from build123d import *

# Parameters (mm, degrees)
SKETCH1_W                     = 32.5
SKETCH1_H                     = 40
BASE_DEPTH                    = 4
SKETCH4_R                     = 0.9
SCANNER_MOUNTING_HOLES_DEPTH  = 44.359687499
SKETCH6_W                     = 6
SKETCH6_H                     = 4.5
SERVO_MOUNTING_PLATFORM_DEPTH = 14
SERVO_MOUNTING_HOLES_REACH    = 51.46
SKETCH7_R                     = 0.9
FILLET1_R                     = 1


with BuildPart() as part:
    # Sketch1 → Base (new body)
    with BuildSketch(Plane(origin=(0, 0, 0), x_dir=(1, 0, 0), z_dir=(0, 1, 0))):
        with Locations((0, 20)):
            Rectangle(SKETCH1_W, SKETCH1_H)
    extrude(amount=BASE_DEPTH)

    # Sketch4 → Scanner Mounting Holes (cut, through all)
    with BuildSketch(Plane.XZ):
        with Locations(Location((-12.35, -6, 0), (0, 0, 270))):
            Circle(SKETCH4_R)
        with Locations(Location((-12.35, -32.4, 0), (0, 0, 270))):
            Circle(SKETCH4_R)
        with Locations(Location((12.35, -32.4, 0), (0, 0, 90))):
            Circle(SKETCH4_R)
        with Locations(Location((12.35, -6, 0), (0, 0, 90))):
            Circle(SKETCH4_R)
    extrude(amount=-SCANNER_MOUNTING_HOLES_DEPTH, mode=Mode.SUBTRACT)

    # Sketch6 → Servo Mounting Platform (add)
    with BuildSketch(Plane.XZ):
        with Locations((-6.25, -6)):
            Rectangle(SKETCH6_W, SKETCH6_H)
        with Locations((-6.25, -33.8)):
            Rectangle(SKETCH6_W, SKETCH6_H)
    extrude(amount=SERVO_MOUNTING_PLATFORM_DEPTH)

    # Sketch7 → Servo Mounting Holes (cut, up to next)
    with BuildSketch(Plane.ZY.offset(9.25), mode=Mode.PRIVATE) as servo_mounting_holes_sk1:
        with Locations((-33.8, -8)):
            Circle(SKETCH7_R)
    servo_mounting_holes_tool1 = extrude(servo_mounting_holes_sk1.sketch, amount=-SERVO_MOUNTING_HOLES_REACH, mode=Mode.PRIVATE) & part.part
    # Sketch7 → Servo Mounting Holes (cut, up to next)
    with BuildSketch(Plane.ZY.offset(9.25), mode=Mode.PRIVATE) as servo_mounting_holes_sk2:
        with Locations((-6, -8)):
            Circle(SKETCH7_R)
    servo_mounting_holes_tool2 = extrude(servo_mounting_holes_sk2.sketch, amount=-SERVO_MOUNTING_HOLES_REACH, mode=Mode.PRIVATE) & part.part
    add(servo_mounting_holes_tool1.solids().sort_by_distance((-9.25, -8, -33.8))[0], mode=Mode.SUBTRACT)
    add(servo_mounting_holes_tool2.solids().sort_by_distance((-9.25, -8, -6))[0], mode=Mode.SUBTRACT)

    # Fillet1
    fillet1_edges = [part.edges().sort_by_distance(p)[0] for p in [
        (16.25, 4, -20),
        (0, 4, -40),
        (-6.25, 0, -8.25),
        (-6.25, 0, -3.75),
        (-9.25, -14, -6),
        (-6.25, -14, -8.25),
        (-3.25, -14, -6),
        (-6.25, -14, -3.75),
        (-6.25, 0, -36.05),
        (-6.25, 0, -31.55),
        (-9.25, -14, -33.8),
        (-6.25, -14, -36.05),
        (-3.25, -14, -33.8),
        (-6.25, -14, -31.55),
        (-16.25, 4, -20),
        (0, 0, -40),
        (16.25, 0, -20),
        (0, 0, 0),
        (-16.25, 0, -20),
        (-16.25, 2, -40),
        (16.25, 2, -40),
        (16.25, 2, 0),
        (-16.25, 2, 0),
        (0, 4, 0),
    ]]
    fillet(fillet1_edges, radius=FILLET1_R)


solid = part.part
Here's how the part is built. I have some questions about the finished solid (model axes, mm). A direction names the side the tool comes from. Give positions to 0.01 mm unless a question says otherwise; leave off trailing zeros. Loops run counter-clockwise (first coordinate to the right, second up) from the corner with the lowest first, then second, coordinate; pieces in that order, holes last. Notation, with made-up numbers: (34, -26.75) -> (93, -26.75) arc R27 cw to (93, -3.75) -> close; hole circle Ø9 at (78, 38). An arc over 180 degrees is marked (long way). Answer as a JSON object with one key per item and string values. Group by question number.
Item 1: Imagine slicing it at D-D on z = -33.8. Write out the boundary of the cut face in (x, y).
Item 2: Imagine slicing it at C-C on x = -12.35. Write out the boundary of the cut face in (y, z).
Item 3: Imagine slicing it at B-B on z = -6. Write out the boundary of the cut face in (x, y).
Item 4: Will these pins go through, and if not, where does the flat tip stop? pin 1 (3 mm diameter, centred on x = 12.35, z = -6, fed in from +Y); pin 2 (3 mm diameter, centred on x = -6, y = -4.5, fed in from +Z); pin 3 (1.8 mm diameter, centred on x = -6, y = -7.5, fed in from -Z); pin 4 (10 mm diameter, centred on y = -11, z = -31, fed in from +X).
Item 5: Imagine slicing it at A-A on y = -4. Write out the boundary of the cut face in (x, z).
Item 6: On a 3-axis mill with a long thin cutter (end or side, diameter ignored), from which of +Z, -Z, +X, -X, +Y, -Y can I reach the whole of each face in a straight line? I mean faces 5 (the flat face through (-6, -7, -8.25)), 6 (the flat face through (-3.25, -6, -6)), 7 (the flat face through (-6, -7, -3.75)), 8 (the cylindrical face through (-15.965, 2.014, -39.699)). Say none if no direction works.
Item 7: Thinking about a two-plate mould opening in Z: for faces 1 (the cylindrical face through (12.3, 2, -6.9)), 2 (the cylindrical face through (-6.3, -8, -34.7)), 3 (the cylindrical face through (-15.965, 3.699, -20.266)), 4 (the flat face through (0, 2, 0)), which applies, pulls with the +Z half, pulls with the -Z half, needs draft (parallel to the pull), parting line crosses it, or undercut?
Item 8: I need wall thicknesses on L1, parallel to X at y = 1.65, z = -6; L2, parallel to Z at x = -3.5, y = -10.5; L3, parallel to Y at x = -3.5, z = -10. Which ranges of each line are inside material? Lowest first, please.
Answer list:
{
 "1": {"outline": "(-16.25, 1) arc R1 ccw to (-15.25, 0) -> (-9.25, 0) -> (-9.25, -7.1) -> (-3.25, -7.1) -> (-3.25, 0) -> (15.25, 0) arc R1 ccw to (16.25, 1) -> (16.25, 3) arc R1 ccw to (15.25, 4) -> (-15.25, 4) arc R1 ccw to (-16.25, 3) -> close; (-9.25, -13) arc R1 ccw to (-8.25, -14) -> (-4.25, -14) arc R1 ccw to (-3.25, -13) -> (-3.25, -8.9) -> (-9.25, -8.9) -> close"},
 "2": {"outline": "(0, -39) arc R1 ccw to (1, -40) -> (3, -40) arc R1 ccw to (4, -39) -> (4, -33.3) -> (0, -33.3) -> close; (0, -31.5) -> (4, -31.5) -> (4, -6.9) -> (0, -6.9) -> close; (0, -5.1) -> (4, -5.1) -> (4, -1) arc R1 ccw to (3, 0) -> (1, 0) arc R1 ccw to (0, -1) -> close"},
 "3": {"outline": "(-16.25, 1) arc R1 ccw to (-15.25, 0) -> (-13.25, 0) -> (-13.25, 4) -> (-15.25, 4) arc R1 ccw to (-16.25, 3) -> close; (-11.45, 0) -> (-9.25, 0) -> (-9.25, -7.1) -> (-3.25, -7.1) -> (-3.25, 0) -> (11.45, 0) -> (11.45, 4) -> (-11.45, 4) -> close; (-9.25, -13) arc R1 ccw to (-8.25, -14) -> (-4.25, -14) arc R1 ccw to (-3.25, -13) -> (-3.25, -8.9) -> (-9.25, -8.9) -> close; (13.25, 0) -> (15.25, 0) arc R1 ccw to (16.25, 1) -> (16.25, 3) arc R1 ccw to (15.25, 4) -> (13.25, 4) -> close"},
 "4": {"pin 1": "stops at y = 4", "pin 2": "stops at z = -3.75", "pin 3": "stops at z = -36.05", "pin 4": "stops at x = -3.25"},
 "5": {"outline": "(-9.25, -36.05) -> (-3.25, -36.05) -> (-3.25, -31.55) -> (-9.25, -31.55) -> close; (-9.25, -8.25) -> (-3.25, -8.25) -> (-3.25, -3.75) -> (-9.25, -3.75) -> close"},
 "6": {"face 5": "+X, -X, -Y", "face 6": "+Z, -Z, +X, -Y", "face 7": "+Z, +X, -X, -Y", "face 8": "-Z, -X, +Y, -Y"},
 "7": {"face 1": "undercut", "face 2": "undercut", "face 3": "needs draft", "face 4": "pulls with the +Z half"},
 "8": {"L1": "x = -16.25 to -13.25, -11.45 to 11.45, 13.25 to 16.25", "L2": "z = -36.05 to -31.55, -8.25 to -3.75", "L3": "y = 0 to 4"}
}
